Autodesk Inventor part; units mm, degrees
ref_plane "YZ Plane" through (0, 0, 0) normal (1, 0, 0) x (0, 1, 0)
ref_plane "XZ Plane" through (0, 0, 0) normal (0, 1, 0) x (-1, 0, 0)
ref_plane "XY Plane" through (0, 0, 0) normal (0, 0, 1) x (1, 0, 0)
sketch "Sketch1" plane through (0, 0, 0) normal (0, 0, 1) x (1, 0, 0)
  line L0 (-12.7, 12.7) -> (12.7, 12.7)
  line L1 (12.7, 12.7) -> (12.7, -12.7)
  line L2 (12.7, -12.7) -> (-12.7, -12.7)
  line L3 (-12.7, -12.7) -> (-12.7, 12.7)
  line L4 (-9.525, -9.525) -> (9.525, -9.525)
  line L5 (9.525, -9.525) -> (9.525, 9.525)
  line L6 (9.525, 9.525) -> (-9.525, 9.525)
  line L7 (-9.525, 9.525) -> (-9.525, -9.525)
  point P0 (0, 0)
  dimension "d0" = 25.4
  dimension "d1" = 25.4
  dimension "d2" = 12.7
  dimension "d3" = 12.7
  dimension "d4" = 3.175
  dimension "d5" = 3.175
  dimension "d6" = 3.175
  dimension "d7" = 3.175
extrude "Extrusion1" add sketch "Sketch1" along normal blind 79.375
sketch "Sketch3" plane through (-12.7, 12.7, 0) normal (0, 1, 0) x (1, 0, 0)
  line L0 (25.4, 0) -> (25.4, -79.375)
  line L1 (0, 0) -> (25.4, 0)
  circle A0 centre (12.7, -66.675) radius 3.175
  point P0 (25.4, -158.75)
  point P1 (12.7, 0)
  dimension "d13" = 66.675
  dimension "d14" = 12.7
  dimension "d15" = 6.35
extrude "Extrusion3" cut sketch "Sketch3" against normal blind 25.4
properties part number "edge frame short"
Source: CAD feature listing. Evaluate the final solid. Frame: model axes, mm. A direction names the side the tool comes from. Coordinates: 2 decimals unless noted, no trailing zeros. Write each loop counter-clockwise with the first axis right and the second up, starting at its lowest first coordinate (ties: lowest second). Pieces come first, ordered by that corner, then holes. Notation, with made-up numbers: (72.5, 42.5) -> (125.5, 42.5) arc R33 cw to (125.5, 74.5) -> close; hole circle Ø1 at (21.25, 21.5). An arc over 180 degrees is marked (long way). Return JSON: item names as keys, results as strings. Group by question number.
1) Section query A-A, the plane y = -0.25. Return loops of the section in (x, z) (3 decimals), plus the area to 3 significant figures.
2) Section query B-B, the plane x = 0. Return loops of the section in (y, z) (3 decimals).
3) Mould query, pull axis Y, two halves, no side actions, for faces 1 (the face through (12.7, 0, 39)), 2 (the face through (0, -12.7, 39)), 3 (the face through (0, -9.525, 39)). Classes: +Y half, -Y half, draft (parallel to the pull), parting line (faces both ways), or undercut.
4) Set-up query: faces 4 (the face through (11, 0, 0)), 5 (the face through (9.525, 0, 39)). Return all of +Z, -Z, +X, -X, +Y, -Y with unobstructed straight access to the full face (end or side cutting, diameter ignored); none if empty.
5) Ray query, line 1 along X through (y, z) = (-7.5, 24) (3 decimals); line 2 along Z through (x, y) = (0, -11.55) (3 decimals). Return the intervals inside material, ascending.
6) Contact query for a flat-ended pin moving along its axis: P1, Ø2, axis at x = -0.5, y = -7.5, coming from the -Z side. Output: stop coordinate, or through.
7) Section query C-C, the plane z = 54. Return loops of the section in (x, y) (3 decimals).
From the geometry:
{
 "1": {"outline": "(-12.7, 0) -> (-9.525, 0) -> (-9.525, 79.375) -> (-12.7, 79.375) -> close; (9.525, 0) -> (12.7, 0) -> (12.7, 79.375) -> (9.525, 79.375) -> close", "area": "504 mm²"},
 "2": {"outline": "(-12.7, 0) -> (-9.525, 0) -> (-9.525, 63.5) -> (-12.7, 63.5) -> close; (-12.7, 69.85) -> (-9.525, 69.85) -> (-9.525, 79.375) -> (-12.7, 79.375) -> close; (9.525, 0) -> (12.7, 0) -> (12.7, 63.5) -> (9.525, 63.5) -> close; (9.525, 69.85) -> (12.7, 69.85) -> (12.7, 79.375) -> (9.525, 79.375) -> close"},
 "3": {"face 1": "draft", "face 2": "-Y half", "face 3": "undercut"},
 "4": {"face 4": "-Z, +X, -X, +Y, -Y", "face 5": "+Z, -Z"},
 "5": {"line 1": "-12.7 to -9.525, 9.525 to 12.7", "line 2": "0 to 63.5, 69.85 to 79.375"},
 "6": {"P1": "through"},
 "7": {"outline": "(-12.7, -12.7) -> (12.7, -12.7) -> (12.7, 12.7) -> (-12.7, 12.7) -> close; hole (-9.525, -9.525) -> (9.525, -9.525) -> (9.525, 9.525) -> (-9.525, 9.525) -> close"}
}
